For this review, take the finished solid that the model builds, in its own axes (mm). Face numbers are marked on the shaded views. Give positions to 0.01 mm unless a question says otherwise; leave off trailing zeros.
from build123d import *

# Parameters (mm, degrees)
SKIZZE1_R                            = 70
AUFSATZ_LINEAR_AUSTRAGEN1_DEPTH      = 0.8
SCHNITT_LINEAR_AUSTRAGEN1_REACH      = 2.8
SKIZZE2_R                            = 2.5
SKIZZE2_R_2                          = 1.5
AUFSATZ_LINEAR_AUSTRAGEN2_DEPTH      = 6
AUFSATZ_LINEAR_AUSTRAGEN2_DEPTH_BACK = 0.8
SKIZZE4_R                            = 1.5
SKIZZE4_R_2                          = 1.410083192
SCHNITT_LINEAR_AUSTRAGEN2_DEPTH      = 1.8
FASE1_SIZE                           = 0.5
SCHNITT_LINEAR_AUSTRAGEN3_REACH      = 8.8
SKIZZE5_R                            = 1.35
SKIZZE6_R                            = 1.6
SCHNITT_LINEAR_AUSTRAGEN4_DEPTH      = 4


with BuildPart() as part:
    # Skizze1 → Aufsatz-Linear austragen1 (new body)
    with BuildSketch(Plane(origin=(0, 0, 0), x_dir=(1, 0, 0), z_dir=(0, 1, 0))):
        Circle(SKIZZE1_R)
    extrude(amount=AUFSATZ_LINEAR_AUSTRAGEN1_DEPTH)

    # Skizze3 → Schnitt-Linear austragen1 (cut, up to next)
    with BuildSketch(Plane.XZ, mode=Mode.PRIVATE) as schnitt_linear_austragen1_sk1:
        with BuildLine():
            Line((6, -10), (0, -10))
            ThreePointArc((0, -10), (-10, 0), (0, 10))
            Line((0, 10), (6, 10))
            ThreePointArc((6, 10), (16, 0), (6, -10))
        make_face()
    schnitt_linear_austragen1_tool1 = extrude(schnitt_linear_austragen1_sk1.sketch, amount=-SCHNITT_LINEAR_AUSTRAGEN1_REACH, mode=Mode.PRIVATE) & part.part
    add(schnitt_linear_austragen1_tool1.solids().sort_by_distance((3, 0, 0))[0], mode=Mode.SUBTRACT)

    # Skizze2 → Aufsatz-Linear austragen2 (add, two sides)
    with BuildSketch(Plane(origin=(0, 0.8, 0), x_dir=(1, 0, 0), z_dir=(0, 1, 0))) as aufsatz_linear_austragen2_sk:
        with Locations((-47.533988615, 40.571841958)):
            Circle(SKIZZE2_R)
        with Locations((-5.293377745, 17.030303573)):
            Circle(SKIZZE2_R)
        with Locations((-47.533988615, -33.027520141)):
            Circle(SKIZZE2_R)
        with Locations((-32.533187453, 16.85488412)):
            Circle(SKIZZE2_R)
        with Locations((-32.533187453, 16.85488412)):
            Circle(SKIZZE2_R_2, mode=Mode.SUBTRACT)
        with Locations((-0.280707317, 46.779952313)):
            Circle(SKIZZE2_R)
        with Locations((-0.280707317, 46.779952313)):
            Circle(SKIZZE2_R_2, mode=Mode.SUBTRACT)
        with Locations((23.260650032, 28.271453094)):
            Circle(SKIZZE2_R)
        with Locations((23.260650032, 28.271453094)):
            Circle(SKIZZE2_R_2, mode=Mode.SUBTRACT)
        with Locations((45.260650032, 28.271453094)):
            Circle(SKIZZE2_R)
        with Locations((45.260650032, 28.271453094)):
            Circle(SKIZZE2_R_2, mode=Mode.SUBTRACT)
        with Locations((45.260650032, -28.428546906)):
            Circle(SKIZZE2_R)
        with Locations((45.260650032, -28.428546906)):
            Circle(SKIZZE2_R_2, mode=Mode.SUBTRACT)
        with Locations((23.260650032, -28.428546906)):
            Circle(SKIZZE2_R)
        with Locations((23.260650032, -28.428546906)):
            Circle(SKIZZE2_R_2, mode=Mode.SUBTRACT)
        with Locations((-0.152992521, -33.940171336)):
            Circle(SKIZZE2_R)
        with Locations((-0.152992521, -33.940171336)):
            Circle(SKIZZE2_R_2, mode=Mode.SUBTRACT)
    extrude(amount=AUFSATZ_LINEAR_AUSTRAGEN2_DEPTH)
    extrude(aufsatz_linear_austragen2_sk.sketch, amount=-AUFSATZ_LINEAR_AUSTRAGEN2_DEPTH_BACK)

    # Skizze4 → Schnitt-Linear austragen2 (cut, through all)
    with BuildSketch(Plane(origin=(0, 0.8, 0), x_dir=(1, 0, 0), z_dir=(0, 1, 0))):
        with Locations((-32.533187453, 16.85488412)):
            Circle(SKIZZE4_R)
        with Locations((23.260650032, 28.271453094)):
            Circle(SKIZZE4_R)
        with Locations((45.260650032, 28.271453094)):
            Circle(SKIZZE4_R)
        with Locations((45.260650032, -28.428546906)):
            Circle(SKIZZE4_R)
        with Locations((23.260650032, -28.428546906)):
            Circle(SKIZZE4_R)
        with Locations((-0.152992521, -33.940171336)):
            Circle(SKIZZE4_R)
        with Locations((-0.280707317, 46.779952313)):
            Circle(SKIZZE4_R_2)
    extrude(amount=-SCHNITT_LINEAR_AUSTRAGEN2_DEPTH, mode=Mode.SUBTRACT)

    # Fase1
    fase1_edges = [part.edges().sort_by_distance(p)[0] for p in [
        (-70, 0, 0),
    ]]
    chamfer(fase1_edges, length=FASE1_SIZE)

    # Skizze5 → Schnitt-Linear austragen3 (cut, up to next)
    with BuildSketch(Plane.XZ, mode=Mode.PRIVATE) as schnitt_linear_austragen3_sk1:
        with Locations((-55, 0)):
            Circle(SKIZZE5_R)
    schnitt_linear_austragen3_tool1 = extrude(schnitt_linear_austragen3_sk1.sketch, amount=-SCHNITT_LINEAR_AUSTRAGEN3_REACH, mode=Mode.PRIVATE) & part.part
    add(schnitt_linear_austragen3_tool1.solids().sort_by_distance((-55, 0, 0))[0], mode=Mode.SUBTRACT)
    # Skizze5 → Schnitt-Linear austragen3 (cut, up to next)
    with BuildSketch(Plane.XZ, mode=Mode.PRIVATE) as schnitt_linear_austragen3_sk2:
        with Locations((55, 0)):
            Circle(SKIZZE5_R)
    schnitt_linear_austragen3_tool2 = extrude(schnitt_linear_austragen3_sk2.sketch, amount=-SCHNITT_LINEAR_AUSTRAGEN3_REACH, mode=Mode.PRIVATE) & part.part
    add(schnitt_linear_austragen3_tool2.solids().sort_by_distance((55, 0, 0))[0], mode=Mode.SUBTRACT)
    # Skizze5 → Schnitt-Linear austragen3 (cut, up to next)
    with BuildSketch(Plane.XZ, mode=Mode.PRIVATE) as schnitt_linear_austragen3_sk3:
        with Locations((0, -55)):
            Circle(SKIZZE5_R)
    schnitt_linear_austragen3_tool3 = extrude(schnitt_linear_austragen3_sk3.sketch, amount=-SCHNITT_LINEAR_AUSTRAGEN3_REACH, mode=Mode.PRIVATE) & part.part
    add(schnitt_linear_austragen3_tool3.solids().sort_by_distance((0, 0, -55))[0], mode=Mode.SUBTRACT)
    # Skizze5 → Schnitt-Linear austragen3 (cut, up to next)
    with BuildSketch(Plane.XZ, mode=Mode.PRIVATE) as schnitt_linear_austragen3_sk4:
        with Locations((0, 55)):
            Circle(SKIZZE5_R)
    schnitt_linear_austragen3_tool4 = extrude(schnitt_linear_austragen3_sk4.sketch, amount=-SCHNITT_LINEAR_AUSTRAGEN3_REACH, mode=Mode.PRIVATE) & part.part
    add(schnitt_linear_austragen3_tool4.solids().sort_by_distance((0, 0, 55))[0], mode=Mode.SUBTRACT)

    # Skizze6 → Schnitt-Linear austragen4 (cut)
    with BuildSketch(Plane(origin=(0, 0, 0), x_dir=(-1, 0, 0), z_dir=(0, -1, 0))):
        with Locations((-10.644187298, 11.605236936)):
            Circle(SKIZZE6_R)
        with Locations((-10.644187298, -11.605236936)):
            Circle(SKIZZE6_R)
    extrude(amount=-SCHNITT_LINEAR_AUSTRAGEN4_DEPTH, mode=Mode.SUBTRACT)


solid = part.part
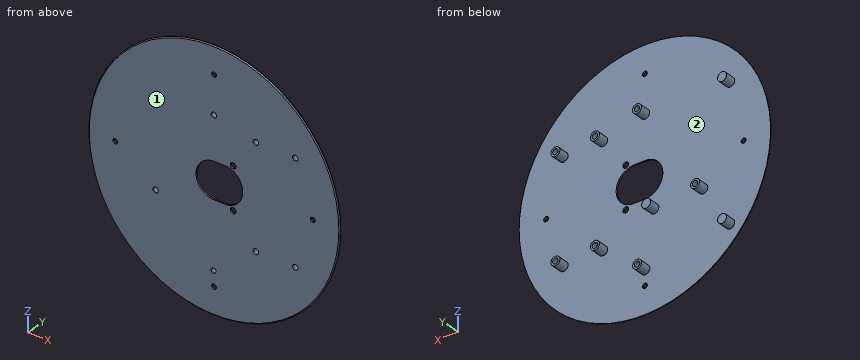
(1) The part is to be moulded in two halves that separate along Y. For the marked faces 1 and 2, say which applies: +Y half, -Y half, draft (parallel to the pull), parting line (faces both ways), or undercut.
(2) Clearance check with flat-ended pins moving along their axes: pin 1 Ø0.9 at (x, z) = (0, -47.5) entering from +Y; pin 2 Ø4.5 at (x, z) = (0, 55) entering from +Y; pin 3 Ø3 at (y, z) = (3.5, -18.5) entering from +X. State where each tip first meets the part, or that it passes through.
(3) For L1, parallel to Z at x = 0, y = 0.4; L2, parallel to X at y = 1.25, z = 28; L3, parallel to X at y = 2, z = -29, list the stretches that pass through material, from the lowest coordinate up.
(4) We need section A-A (y = 4). Count the separate pieces of the cut face and the enclosed holes in it, and give its area (3 significant figures).
The answers:
1. face 1: -Y half
1. face 2: +Y half
2. pin 1: passes through
2. pin 2: stops at y = 0.8
2. pin 3: stops at x = -2.79
3. L1: z = -69.9 to -56.35, -53.65 to -48.16, -45.4 to -10, 10 to 32.45, 35.43 to 53.65, 56.35 to 69.9
3. L2: x = 20.8 to 21.82, 24.7 to 25.72, 42.8 to 43.82, 46.7 to 47.72
3. L3: x = 20.87 to 21.95, 24.57 to 25.65, 42.87 to 43.95, 46.57 to 47.65
4. separate pieces: 10
4. enclosed holes: 7
4. area: 147 mm2
